from build123d import *

# Parameters (mm, degrees)
CROQUIS1_W              = 45.6
CROQUIS1_H              = 24.9
SALIENTE_EXTRUIR1_DEPTH = 2.5
SALIENTE_EXTRUIR1_TAPER = 3
CROQUIS2_W              = 51.6
CROQUIS2_H              = 30.9
SALIENTE_EXTRUIR2_DEPTH = 2
REDONDEO1_R             = 3
CROQUIS3_R              = 2.75
CROQUIS3_W              = 8
CROQUIS3_H              = 3
CROQUIS3_W_2            = 5.5
CROQUIS3_H_2            = 9
CORTAR_EXTRUIR1_DEPTH   = 5
VACIADO1_START          = -10.447255308
VACIADO1_OUTLINE_W      = 2.9
VACIADO1_OUTLINE_H      = 2.5
VACIADO1_DEPTH          = 20.894510616
VACIADO1_2_OUTLINE_W    = 12
VACIADO1_2_OUTLINE_H    = 2.5
VACIADO1_2_DEPTH        = 12.897255308
VACIADO1_START_2        = 4.05
VACIADO1_3_OUTLINE_W    = 9.5
VACIADO1_3_OUTLINE_H    = 2.5
VACIADO1_3_DEPTH        = 6.397255308
VACIADO1_4_OUTLINE_W    = 9.5
VACIADO1_4_OUTLINE_H    = 2.5
VACIADO1_4_DEPTH        = 1.497255308
VACIADO1_START_3        = 9.45
VACIADO1_5_OUTLINE_W    = 12
VACIADO1_5_OUTLINE_H    = 2.5
VACIADO1_5_DEPTH        = 0.997255308
VACIADO1_START_4        = -7.073070686
VACIADO1_6_DEPTH        = 29.742051238
VACIADO1_START_5        = -22.668980552
VACIADO1_7_DEPTH        = 10.789333394
VACIADO1_START_6        = -12.0000001
VACIADO1_8_DEPTH        = 5.350388625
VACIADO1_9_DEPTH        = 2.5
CROQUIS4_W              = 1.002744692
CROQUIS4_H              = 20.63247172
CORTAR_EXTRUIR2_DEPTH   = 2.5
CROQUIS6_W              = 9.5
CROQUIS6_H              = 13
CROQUIS6_W_2            = 5.5
CROQUIS6_H_2            = 9
SALIENTE_EXTRUIR3_DEPTH = 5
CROQUIS7_W              = 15.957634565
CROQUIS7_H              = 9.76050456
CORTAR_EXTRUIR3_DEPTH   = 2.5


with BuildPart() as part:
    # Croquis1 → Saliente-Extruir1 (new body)
    with BuildSketch(Plane(origin=(0, 0, 0), x_dir=(1, 0, 0), z_dir=(0, 1, 0))):
        Rectangle(CROQUIS1_W, CROQUIS1_H)
    extrude(amount=SALIENTE_EXTRUIR1_DEPTH, taper=SALIENTE_EXTRUIR1_TAPER)

    # Croquis2 → Saliente-Extruir2 (add)
    with BuildSketch(Plane.XZ):
        Rectangle(CROQUIS2_W, CROQUIS2_H)
    extrude(amount=SALIENTE_EXTRUIR2_DEPTH)

    # Redondeo1
    redondeo1_edges = [part.edges().sort_by_distance(p)[0] for p in [
        (-25.8, -1, 15.45),
        (-25.8, -1, -15.45),
        (25.8, -1, -15.45),
        (25.8, -1, 15.45),
    ]]
    fillet(redondeo1_edges, radius=REDONDEO1_R)

    # Croquis3 → Cortar-Extruir1 (cut)
    with BuildSketch(Plane.XZ.offset(2)):
        with Locations(Location((-9.25, -8.1, 0), (0, 0, 270))):
            Circle(CROQUIS3_R)
        with Locations((-4.1, 5.95)):
            Rectangle(CROQUIS3_W, CROQUIS3_H)
        with Locations((9.55, -2.45)):
            Rectangle(CROQUIS3_W_2, CROQUIS3_H_2)
    extrude(amount=-CORTAR_EXTRUIR1_DEPTH, mode=Mode.SUBTRACT)

    # Vaciado1: read off the stored shape, not the designer's step
    # Vaciado1 outline → Vaciado1 (cut)
    with BuildSketch(Plane.XY.offset(VACIADO1_START)):
        Polygon((-20.66623586, 2.5), (-20.797255308, 0), (-10.1, 0), (-10.1, 2.5), align=None)
        with Locations((3.35, 1.25)):
            Rectangle(VACIADO1_OUTLINE_W, VACIADO1_OUTLINE_H)
        Polygon((14.3, 2.5), (14.3, 0), (20.797255308, 0), (20.66623586, 2.5), align=None)
    extrude(amount=VACIADO1_DEPTH, mode=Mode.SUBTRACT)

    # Vaciado1 2 outline → Vaciado1 2 (cut)
    with BuildSketch(Plane.XY.offset(VACIADO1_START)):
        with Locations((-4.1, 1.25)):
            Rectangle(VACIADO1_2_OUTLINE_W, VACIADO1_2_OUTLINE_H)
    extrude(amount=VACIADO1_2_DEPTH, mode=Mode.SUBTRACT)

    # Vaciado1 3 outline → Vaciado1 3 (cut)
    with BuildSketch(Plane.XY.offset(VACIADO1_START_2)):
        with Locations((9.55, 1.25)):
            Rectangle(VACIADO1_3_OUTLINE_W, VACIADO1_3_OUTLINE_H)
    extrude(amount=VACIADO1_3_DEPTH, mode=Mode.SUBTRACT)

    # Vaciado1 4 outline → Vaciado1 4 (cut)
    with BuildSketch(Plane.XY.offset(VACIADO1_START)):
        with Locations((9.55, 1.25)):
            Rectangle(VACIADO1_4_OUTLINE_W, VACIADO1_4_OUTLINE_H)
    extrude(amount=VACIADO1_4_DEPTH, mode=Mode.SUBTRACT)

    # Vaciado1 5 outline → Vaciado1 5 (cut)
    with BuildSketch(Plane.XY.offset(VACIADO1_START_3)):
        with Locations((-4.1, 1.25)):
            Rectangle(VACIADO1_5_OUTLINE_W, VACIADO1_5_OUTLINE_H)
    extrude(amount=VACIADO1_5_DEPTH, mode=Mode.SUBTRACT)

    # Vaciado1 6 outline → Vaciado1 6 (add)
    with BuildSketch(Plane.YZ.offset(VACIADO1_START_4)):
        Polygon((0, -10.447255308), (2.5, -10.447255308), (2.5, -10.31623586), align=None)
        Polygon((0, 10.447255308), (2.5, 10.31623586), (2.5, 10.447255308), align=None)
    extrude(amount=VACIADO1_6_DEPTH)

    # Vaciado1 7 outline → Vaciado1 7 (add)
    with BuildSketch(Plane.YZ.offset(VACIADO1_START_5)):
        Polygon((0, -10.447255308), (2.5, -10.447255308), (2.5, -10.31623586), align=None)
        Polygon((0, 10.447255308), (2.5, 10.31623586), (2.5, 10.447255308), align=None)
    extrude(amount=VACIADO1_7_DEPTH)

    # Vaciado1 8 outline → Vaciado1 8 (add)
    with BuildSketch(Plane.YZ.offset(VACIADO1_START_6)):
        Polygon((0, 10.447255308), (2.5, 10.31623586), (2.5, 10.447255308), align=None)
    extrude(amount=VACIADO1_8_DEPTH)

    # Vaciado1 9 outline → Vaciado1 9 (add)
    with BuildSketch(Plane(origin=(0, 0, 0), x_dir=(1, 0, 0), z_dir=(0, 1, 0))):
        with BuildLine():
            ThreePointArc((-7.817208138, 10.447255308), (-9.25, 5.35), (-10.682791862, 10.447255308))
            Line((-10.682791862, 10.447255308), (-13.379514804, 10.447255308))
            ThreePointArc((-13.379514804, 10.447255308), (-9.25, 3.35), (-5.120485196, 10.447255308))
            Line((-5.120485196, 10.447255308), (-7.817208138, 10.447255308))
        make_face()
    extrude(amount=VACIADO1_9_DEPTH)

    # Croquis4 → Cortar-Extruir2 (cut)
    with BuildSketch(Plane(origin=(0, 2.5, 0), x_dir=(1, 0, 0), z_dir=(0, 1, 0))):
        with Locations((-21.167608206, 0)):
            Rectangle(CROQUIS4_W, CROQUIS4_H)
    extrude(amount=-CORTAR_EXTRUIR2_DEPTH, mode=Mode.SUBTRACT)

    # Croquis6 → Saliente-Extruir3 (add)
    with BuildSketch(Plane(origin=(0, 2.5, 0), x_dir=(1, 0, 0), z_dir=(0, 1, 0))):
        with Locations((9.55, 2.45)):
            Rectangle(CROQUIS6_W, CROQUIS6_H)
        with Locations((9.55, 2.45)):
            Rectangle(CROQUIS6_W_2, CROQUIS6_H_2, mode=Mode.SUBTRACT)
    extrude(amount=SALIENTE_EXTRUIR3_DEPTH)

    # Croquis7 → Cortar-Extruir3 (cut)
    with BuildSketch(Plane(origin=(0, 2.5, 0), x_dir=(1, 0, 0), z_dir=(0, 1, 0))):
        with Locations((-9.332505864, 5.43598358)):
            Rectangle(CROQUIS7_W, CROQUIS7_H)
    extrude(amount=-CORTAR_EXTRUIR3_DEPTH, mode=Mode.SUBTRACT)


solid = part.part
Model file for the job. Use its own axes, mm. A direction names the side the tool comes from. Round coordinates to 2 decimals unless told otherwise and drop trailing zeros. Order: outer loops, then holes, each group sorted by start corner. A loop starts at its lowest first (then second) coordinate and runs counter-clockwise, first axis right, second up.
(1) Band-saw the part on C-C (z = 13.5). List the corners of the cut face in (x, y), then the cut area to 3 significant figures.
(2) Band-saw the part on A-A (y = 3.75). List the corners of the cut face in (x, z), then the cut area to 3 significant figures.
(3) Pin check, flat tips, straight feed: pin 1 (4 mm diameter, centred on x = 10.5, y = 4, fed in from -Z); pin 2 (5 mm diameter, centred on y = 6.5, z = 0.5, fed in from -X); pin 3 (1.2 mm diameter, centred on x = -6, y = 2, fed in from +Z). Stop position of each tip, or through.
(4) 3-axis set-ups, long thin cutter, end or side, ignore diameter. For faces 4 (the face through (-21.669, 1, 0)), 5 (the face through (-8.1, 0, 6)), 6 (the face through (24.9, -1.01, 14.59)): which of +Z, -Z, +X, -X, +Y, -Y reach the whole face in a straight line?
(5) Drill centre lines: line 1 (X direction, y = 1.35, z = -8.1); line 2 (X direction, y = 5.75, z = -3.5); line 3 (Z direction, x = -9.25, y = -0.35). Where is each one in solid material? Low to high.
(6) Band-saw the part on B-B (y = 1). Give the number of separate pieces and of enclosed holes in the cut face, then the cut area to 3 significant figures.
(7) Pull direction Y, two halves, no side cores. Call faces 1 (the face through (-0.291, 1.232, 10.383)), 2 (the face through (6.8, 3, -2)), 3 (the face through (0, -2, 0)): released by +Y, released by -Y, zero draft, split by the parting line, or undercut.
Verdict:
1. outline: (-25.61, -2) - (25.61, -2) - (25.61, 0) - (-25.61, 0) - close
1. area: 102 mm2
2. outline: (4.8, -8.95) - (14.3, -8.95) - (14.3, 4.05) - (4.8, 4.05) - close; hole (6.8, -6.95) - (12.3, -6.95) - (12.3, 2.05) - (6.8, 2.05) - close
2. area: 74.0 mm2
3. pin 1: stops at z = -12.35
3. pin 2: stops at x = 4.8
3. pin 3: stops at z = 12.38
4. face 4: +Y
4. face 5: +Y, -Y
4. face 6: +Z, +X, +Y, -Y
5. line 1: x = -22.73 to -21.67, 4.8 to 14.3, 20.73 to 22.73
5. line 2: x = 4.8 to 6.8, 12.3 to 14.3
5. line 3: z = -15.45 to -10.85, -5.35 to 15.45
6. separate pieces: 3
6. enclosed holes: 3
6. area: 380 mm2
7. face 1: undercut
7. face 2: zero draft
7. face 3: released by -Y
